Can you work these out from the model? Positions are in its coordinate system, mm. Face numbers are marked on the shaded views. Give positions to 0.01 mm unless a question says otherwise; leave off trailing zeros. Order: outer loops, then holes, each group sorted by start corner. A loop starts at its lowest first (then second) coordinate and runs counter-clockwise, first axis right, second up.
```python
from build123d import *

# Parameters (mm, degrees)
F0_W      = 99.06
F0_H      = 80.01
F1_DEPTH  = 8.89
F3_W      = 2.54
F3_H      = 25.4
F4_DEPTH  = 1.27
F2_W      = 2.54
F2_H      = 25.4
F5_DEPTH  = 1.27
F6_W      = 85.09
F6_H      = 6.35
F7_DEPTH  = 3.81
F8_W      = 99.06
F8_H      = 2.413
F9_DEPTH  = 6.35
F10_DEPTH = 15.24


# Not quite as in the source:
# - a feature names something its author has since deleted; it is built from what else it names


with BuildPart() as f1:
    # F0 (on Front) → F1 (new body)
    with BuildSketch(Plane.XZ):
        Rectangle(F0_W, F0_H)
    extrude(amount=F1_DEPTH)

    # F3 (on face) → F4 (join)
    with BuildSketch(Plane(origin=(-49.53, 0, 0), x_dir=(0, -1, 0), z_dir=(-1, 0, 0))):
        with Locations((7.62, 27.305)):
            Rectangle(F3_W, F3_H)
    extrude(amount=F4_DEPTH)

    # F2 (on face) → F5 (join)
    with BuildSketch(Plane.YZ.offset(49.53)):
        with Locations((-7.62, 27.305)):
            Rectangle(F2_W, F2_H)
    extrude(amount=F5_DEPTH)

    # F6 (on face) → F7 (join)
    with BuildSketch(Plane(origin=(0, 0, -40.005), x_dir=(1, 0, 0), z_dir=(0, 0, -1))):
        with Locations((-6.985, 12.065)):
            Rectangle(F6_W, F6_H)
        Polygon((35.56, 8.89), (-49.53, 8.89), (-49.53, 0), (49.53, 0), (49.53, 8.89), align=None)
    extrude(amount=F7_DEPTH)

    # F8 (on face) → F9 (join)
    with BuildSketch(Plane.XZ.offset(8.89)):
        with Locations((0, 38.7985)):
            Rectangle(F8_W, F8_H)
    extrude(amount=F9_DEPTH)

    # F10 (add): a face of the model
    f10_faces = [f1.faces().sort_by_distance(p)[0] for p in [
        (35.56, -12.065, -41.91),
    ]]
    extrude(f10_faces, amount=F10_DEPTH)


solid = f1.part
```
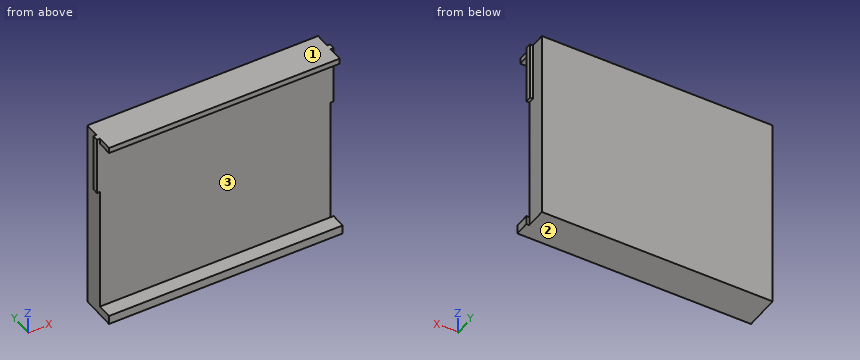
1) Suppose I cut it at C-C (z = 27.5). Please give me the cut outline in (x, y), and give its area (3 significant figures).
2) We'd pull the mould along Z, two halves only. Please class the marked faces 1, 2 and 3: +Z half, -Z half, draft (parallel to the pull), parting line (faces both ways), or undercut.
3) I'm going to push flat-ended pins straight in: pin 1 Ø0.7 at (y, z) = (-11.5, 39) entering from +X; pin 2 Ø24 at (x, z) = (-15, -18.5) entering from -Y; pin 3 Ø1 at (x, z) = (50.5, 25.5) entering from +Y; pin 4 Ø6 at (y, z) = (-12, 16.5) entering from +X. Where does each tip first touch, or does it pass through?
4) Suppose I cut it at A-A (y = -13). Please give me the cut outline in (x, z) (3 decimals).
5) Suppose I cut it at B-B (y = -7.5). Please give me the cut outline in (x, z) (3 decimals), and give its area (3 significant figures).
6) Suppose I cut it at D-D (z = -7). Please give me the cut outline in (x, y), and give its area (3 significant figures).
7) If I drill on line 1 (Z direction, x = 8, y = -10) (3 decimals); line 2 (Y direction, x = 3, z = -29); line 3 (X direction, y = -2.75, z = -10.5), over which ranges is the centre line in solid material (lowest first)?
Results:
1. outline: (-50.8, -8.89) - (50.8, -8.89) - (50.8, -6.35) - (49.53, -6.35) - (49.53, 0) - (-49.53, 0) - (-49.53, -6.35) - (-50.8, -6.35) - close
1. area: 887 mm2
2. face 1: +Z half
2. face 2: -Z half
2. face 3: undercut
3. pin 1: stops at x = 49.53
3. pin 2: stops at y = -8.89
3. pin 3: stops at y = -6.35
3. pin 4: passes through
4. outline: (-49.53, -43.815) - (50.8, -43.815) - (50.8, -40.005) - (-49.53, -40.005) - close; (-49.53, 37.592) - (49.53, 37.592) - (49.53, 40.005) - (-49.53, 40.005) - close
5. outline: (-50.8, 14.605) - (-49.53, 14.605) - (-49.53, -43.815) - (49.53, -43.815) - (49.53, 14.605) - (50.8, 14.605) - (50.8, 40.005) - (-50.8, 40.005) - close
5. area: 8,370 mm2
6. outline: (-49.53, -8.89) - (49.53, -8.89) - (49.53, 0) - (-49.53, 0) - close
6. area: 881 mm2
7. line 1: z = -43.815 to -40.005, 37.592 to 40.005
7. line 2: y = -8.89 to 0
7. line 3: x = -49.53 to 49.53
